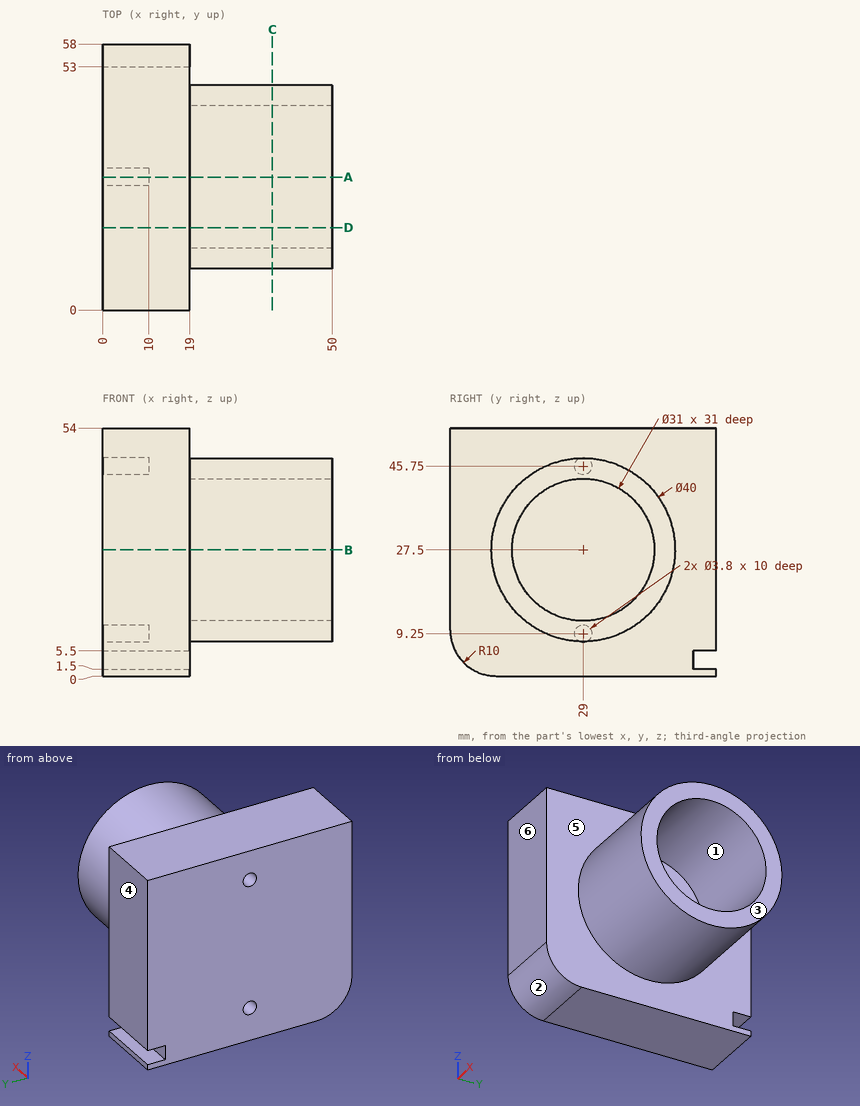
Design review of the part shown in the three views and the two pictorial views. Dimensions are in mm from the part's minimum x, y and z. A direction names the side the tool comes from. Coordinates: 2 decimals unless noted, no trailing zeros. Write each loop counter-clockwise with the first axis right and the second up, starting at its lowest first coordinate (ties: lowest second). Pieces come first, ordered by that corner, then holes. Notation, with made-up numbers: (53, 82.5) - (71, 82.5) arc R26 ccw to (71, 101.5) - close; hole circle Ø10 at (18.5, -21). An arc over 180 degrees is marked (long way). Write item = value, one per line.
(1) Mouldability with a two-part tool opening along Y and no side actions: class the marked faces 1, 2, 3 and 4 as pulls with the +Y half, pulls with the -Y half, needs draft (parallel to the pull), parting line crosses it, or undercut.
Result sheet:
face_1 = undercut
face_2 = pulls with the -Y half
face_3 = needs draft
face_4 = pulls with the +Y half
(2) Consider section A-A, the plane y = 29. Give the boundary of the cut face in (x, z).
Result sheet:
outline = (0, 0) - (19, 0) - (19, 7.5) - (50, 7.5) - (50, 12) - (19, 12) - (19, 43) - (50, 43) - (50, 47.5) - (19, 47.5) - (19, 54) - (0, 54) - (0, 47.65) - (10, 47.65) - (10, 43.85) - (0, 43.85) - (0, 11.15) - (10, 11.15) - (10, 7.35) - (0, 7.35) - close
(3) For P1, Ø1.2, axis at x = 9.5, z = 3, coming from the +Y side; P2, Ø10, axis at x = 34.5, z = 29, coming from the +Y side; P3, Ø12, axis at y = 18.5, z = 36.5, coming from the -X side; P4, Ø3, axis at y = 46.5, z = 44, coming from the +X side, all flat-tipped, find the tip position at first contact; note any pin that passes through.
Result sheet:
P1 = 53
P2 = 49
P3 = 0
P4 = 19
(4) Consider section B-B, the plane z = 27.5. Give the boundary of the cut face in (x, y).
Result sheet:
outline = (0, 0) - (19, 0) - (19, 9) - (50, 9) - (50, 13.5) - (19, 13.5) - (19, 44.5) - (50, 44.5) - (50, 49) - (19, 49) - (19, 58) - (0, 58) - close
(5) Machinability: for the marked faces 5 and 6, which of the approach directions +Z, -Z, +X, -X, +Y, -Y give a long, thin tool a straight path to every point of the face, cutting with its end or side? Answer none if there is none.
Result sheet:
face_5 = +X
face_6 = +Z, -Z, +X, -X, -Y
(6) For line 1 (Y direction, x = 2.75, z = 45.75); line 2 (Y direction, x = 33, z = 27); line 3 (Z direction, x = 45, y = 29.5), list the stretches that pass through material, from the lowest coordinate up. Write a range as [from, to].
Result sheet:
line_1 = [0, 27.1], [30.9, 58]
line_2 = [9.01, 13.51], [44.49, 48.99]
line_3 = [7.51, 12.01], [42.99, 47.49]
(7) Consider section C-C, the plane x = 37. Give the boundary of the cut face in (y, z).
Result sheet:
outline = circle Ø40 at (29, 27.5); hole circle Ø31 at (29, 27.5)
(8) Consider section D-D, the plane y = 18. Give the boundary of the cut face in (x, z), then the cut area to 3 significant figures.
Result sheet:
outline = (0, 0) - (19, 0) - (19, 10.8) - (50, 10.8) - (50, 16.58) - (19, 16.58) - (19, 38.42) - (50, 38.42) - (50, 44.2) - (19, 44.2) - (19, 54) - (0, 54) - close
area = 1,380 mm^2
